Work out the finished part from the listing and answer in its coordinate system (mm). Round coordinates to 2 decimals unless told otherwise and drop trailing zeros. Loops run counter-clockwise (first coordinate to the right, second up) from the corner with the lowest first, then second, coordinate; pieces in that order, holes last. Notation, with made-up numbers: (79, 85.25) - (137, 85.25) arc R18 cw to (137, 120.25) - close; hole circle Ø3 at (-7, -27.75). An arc over 180 degrees is marked (long way). Answer as CSV lines item,"result". Start each with the question number.
Q1. Section C-C on z = 64 is taken. Write down the section's boundary in (x, y), then the cut area to 3 significant figures.
Q2. The mould has two halves that part along X. Classify faces 1 (the face through (-7.2, 32.4, 36.48)), 2 (the face through (32.895, -10.359, 31.41)), 3 (the face through (0, 0, 0)), 4 (the face through (0, 0, 12)): +X half, -X half, draft (parallel to the pull), parting line (faces both ways), or undercut.
Q3. Each of these flat-tipped pins is pushed along its axis until it touches: pin 1 Ø10 at (x, z) = (-3.5, 40) entering from +Y; pin 2 Ø5 at (x, z) = (-8.5, 12) entering from +Y; pin 3 Ø6 at (y, z) = (-24, 50.5) entering from -X. Where does it stop, or does it pass through?
Q4. Section D-D on z = 19.5 is taken. Write down the section's boundary in (x, y), then the cut area to 3 significant figures.
Q5. Straight lines are drawn through the part: L1, parallel to Y at x = 7.5, z = 17; L2, parallel to Y at x = 24.5, z = 60; L3, parallel to X at y = -16, z = 64. For each, find the intervals that lie inside material, in ascending order. Write a range as [from, to].
Q6. Section A-A on y = 0 is taken. Write down the section's boundary in (x, z), then the cut area to 3 significant figures.
```python
from build123d import *


with BuildPart() as f1:
    # F0 (on Front) → F1 (revolve)
    with BuildSketch(Plane.XZ):
        with BuildLine():
            Line((25.357504, 12), (0, 12))
            Line((0, 12), (0, 0))
            Line((0, 0), (23.061637, 0))
            ThreePointArc((23.061637, 0), (28.303251, 1.956368), (30.981233, 6.868629))
            Line((30.981233, 6.868629), (39.83694, 68.858579))
            ThreePointArc((39.83694, 68.858579), (38.988412, 69.989949), (37.857041, 69.141421))
            Line((37.857041, 69.141421), (30.307251, 16.292893))
            ThreePointArc((30.307251, 16.292893), (28.633512, 13.22273), (25.357504, 12))
        make_face()
    revolve(axis=Axis((0, 0, 6), (0, 0, -1)))


solid = f1.part
```
Findings:
1,outline,"circle Ø78.29 at (0, 0); hole circle Ø74.25 at (0, 0)"
1,area,"484 mm^2"
2,face 1,"undercut"
2,face 2,"parting line"
2,face 3,"draft"
2,face 4,"undercut"
3,pin 1,"stops at y = 36.34"
3,pin 2,"stops at y = 31.26"
3,pin 3,"stops at x = -30.79"
4,outline,"circle Ø65.57 at (0, 0); hole circle Ø61.53 at (0, 0)"
4,area,"403 mm^2"
5,L1,"y = [-31.55, -29.47], [29.47, 31.55]"
5,L2,"y = [-29.79, -27.12], [27.12, 29.79]"
5,L3,"x = [-35.72, -33.5], [33.5, 35.72]"
6,outline,"(-39.84, 68.86) - (-30.98, 6.87) arc R8 ccw to (-23.06, 0) - (23.06, 0) arc R8 ccw to (30.98, 6.87) - (39.84, 68.86) arc R1 ccw to (37.86, 69.14) - (30.31, 16.29) arc R5 cw to (25.36, 12) - (-25.36, 12) arc R5 cw to (-30.31, 16.29) - (-37.86, 69.14) arc R1 ccw to start"
6,area,"962 mm^2"
